```python
from build123d import *

# Parameters (mm, degrees)
SKETCH_2_W          = 50
SKETCH_2_H          = 50
SKETCH_2_R          = 2.6
EXTRUDE_1_DEPTH     = 2
SKETCH_3_W          = 50
SKETCH_3_H          = 50
SKETCH_3_R          = 5.15
SKETCH_3_R_2        = 2.6
EXTRUDE_2_DEPTH     = 5.2
SKETCH_4_R          = 2.1
CUT_EXTRUDE_1_DEPTH = 10
CUT_EXTRUDE_2_DEPTH = 3.5
FILLET_1_R          = 6.17
FILLET_2_R          = 6.17
FILLET_3_R          = 6.17
FILLET_4_R          = 6.17


with BuildPart() as part:
    # 스케치2 → 보스-돌출1 (new body)
    with BuildSketch(Plane(origin=(0, 0, 0), x_dir=(1, 0, 0), z_dir=(0, 1, 0))):
        Rectangle(SKETCH_2_W, SKETCH_2_H)
        Circle(SKETCH_2_R, mode=Mode.SUBTRACT)
        with Locations((10, 0)):
            Circle(SKETCH_2_R, mode=Mode.SUBTRACT)
        with Locations((0, -10)):
            Circle(SKETCH_2_R, mode=Mode.SUBTRACT)
        with Locations((-10, 0)):
            Circle(SKETCH_2_R, mode=Mode.SUBTRACT)
        with Locations((0, 10)):
            Circle(SKETCH_2_R, mode=Mode.SUBTRACT)
    extrude(amount=EXTRUDE_1_DEPTH)

    # 스케치3 → 보스-돌출2 (add)
    with BuildSketch(Plane(origin=(0, 2, 0), x_dir=(1, 0, 0), z_dir=(0, 1, 0))):
        Rectangle(SKETCH_3_W, SKETCH_3_H)
        with Locations((0, -10)):
            Circle(SKETCH_3_R, mode=Mode.SUBTRACT)
        with Locations((-10, 0)):
            Circle(SKETCH_3_R, mode=Mode.SUBTRACT)
        Circle(SKETCH_3_R_2, mode=Mode.SUBTRACT)
        with Locations((10, 0)):
            Circle(SKETCH_3_R, mode=Mode.SUBTRACT)
        with Locations((0, 10)):
            Circle(SKETCH_3_R, mode=Mode.SUBTRACT)
    extrude(amount=EXTRUDE_2_DEPTH)

    # 스케치4 → 컷-돌출1 (cut)
    with BuildSketch(Plane(origin=(0, 7.2, 0), x_dir=(1, 0, 0), z_dir=(0, 1, 0))):
        with Locations((20, 0)):
            Circle(SKETCH_4_R)
        with Locations((0, 20)):
            Circle(SKETCH_4_R)
        with Locations((-20, 0)):
            Circle(SKETCH_4_R)
    extrude(amount=-CUT_EXTRUDE_1_DEPTH, mode=Mode.SUBTRACT)

    # 스케치6 → 컷-돌출2 (cut)
    with BuildSketch(Plane.XZ):
        Polygon((-16.45, -2.049593456), (-16.45, 2.049593456), (-20, 4.099186911), (-23.55, 2.049593456), (-23.55, -2.049593456), (-20, -4.099186911), align=None)
        Polygon((2.049593456, -16.45), (-2.049593456, -16.45), (-4.099186911, -20), (-2.049593456, -23.55), (2.049593456, -23.55), (4.099186911, -20), align=None)
        Polygon((16.45, 2.049593456), (16.45, -2.049593456), (20, -4.099186911), (23.55, -2.049593456), (23.55, 2.049593456), (20, 4.099186911), align=None)
    extrude(amount=-CUT_EXTRUDE_2_DEPTH, mode=Mode.SUBTRACT)

    # 필렛1
    fillet_1_edges = [part.edges().sort_by_distance(p)[0] for p in [
        (25, 3.6, -25),
    ]]
    fillet(fillet_1_edges, radius=FILLET_1_R)

    # 필렛2
    fillet_2_edges = [part.edges().sort_by_distance(p)[0] for p in [
        (25, 3.6, 25),
    ]]
    fillet(fillet_2_edges, radius=FILLET_2_R)

    # 필렛3
    fillet_3_edges = [part.edges().sort_by_distance(p)[0] for p in [
        (-25, 3.6, 25),
    ]]
    fillet(fillet_3_edges, radius=FILLET_3_R)

    # 필렛4
    fillet_4_edges = [part.edges().sort_by_distance(p)[0] for p in [
        (-25, 3.6, -25),
    ]]
    fillet(fillet_4_edges, radius=FILLET_4_R)


solid = part.part
```
Build history of the part. All positions in model axes, mm. A direction names the side the tool comes from. Coordinates: 2 decimals unless noted, no trailing zeros. Order: outer loops, then holes, each group sorted by start corner. A loop starts at its lowest first (then second) coordinate and runs counter-clockwise, first axis right, second up. Notation, with made-up numbers: M -15,86.5 L 24,86.5 A8 cw 24,101.5 Z; hole C -7,59 d8. An arc over 180 degrees is marked long. One line per question, with ' | ' between items. Start each with the question number.
1. Flat gauge pins, fed straight in: P1, Ø4, axis at x = 20, z = 0, coming from the -Y side; P2, Ø3, axis at x = -2, z = 9.5, coming from the +Y side. Where does each tip first touch, or does it go through?
2. Tool access for faces 1 (the face through (21.8, 1.73, 3.06)), 2 (the face through (-5.09, 4.56, -1.55)), 3 (the face through (-0.338, 3.55, -2.578)): list every direction of +Z, -Z, +X, -X, +Y, -Y with a clear straight run to the whole face (end or side of a thin tool).
3. Cut at B-B (y = 5.5). Count the separate pieces of the cut face and the enclosed holes in it, plus the area to 3 significant figures.
4. Wall check: line 1 along X through (y, z) = (4.5, 0); line 2 along Z through (x, y) = (10, 4.95). Give the ranges that are in metal, low to high. Write a range as [from, to].
5. Cut at A-A (z = -10). Write the cut outline in (x, y), plus the area to 3 significant figures.
6. Cut at C-C (x = -10). Write the cut outline in (y, z), plus the area to 3 significant figures.
7. Mould opens along X. For faces 4 (the face through (0, 2, -23.55)), 5 (the face through (0, 4, -25)), 6 (the face through (18.2, 1.73, -3.06)), 7 (the face through (25, 4, 0)) say: +X half, -X half, draft (parallel to the pull), parting line (faces both ways), or undercut.
The answers:
1) P1: passes through | P2: stops at y = 2
2) face 1: -Y | face 2: +Y | face 3: +Y, -Y
3) separate pieces: 1 | enclosed holes: 8 | area: 2,070 mm2
4) line 1: x = [-25, -22.1], [-17.9, -15.15], [-4.85, -2.6], [2.6, 4.85], [15.15, 17.9], [22.1, 25] | line 2: z = [-25, -5.15], [5.15, 25]
5) outline: M -25,0 L -2.6,0 L -2.6,2 L -5.15,2 L -5.15,7.2 L -25,7.2 Z; M 2.6,0 L 25,0 L 25,7.2 L 5.15,7.2 L 5.15,2 L 2.6,2 Z | area: 296 mm2
6) outline: M 0,-25 L 7.2,-25 L 7.2,-5.15 L 2,-5.15 L 2,-2.6 L 0,-2.6 Z; M 0,2.6 L 2,2.6 L 2,5.15 L 7.2,5.15 L 7.2,25 L 0,25 Z | area: 296 mm2
7) face 4: undercut | face 5: draft | face 6: undercut | face 7: +X half
